CAD build for the part. Positions are in the model's coordinates, mm. Round coordinates to 2 decimals unless told otherwise and drop trailing zeros. Order: outer loops, then holes, each group sorted by start corner. A loop starts at its lowest first (then second) coordinate and runs counter-clockwise, first axis right, second up. Notation, with made-up numbers: (82, -24.75) -> (104, -24.75) arc R24 cw to (104, -1.75) -> close; hole circle Ø4 at (42.25, -7). An arc over 180 degrees is marked (long way). Return JSON: item names as keys, results as strings. Group by question number.
Q1. Cut at A-A (y = -1.75). Write the cut outline in (x, z).
Q2. Flat gauge pins, fed straight in: pin 1 (1 mm diameter, centred on x = -24.5, y = -3, fed in from +Z); pin 2 (3 mm diameter, centred on y = -1, z = -44, fed in from +X); pin 3 (2 mm diameter, centred on y = -1.5, z = -33.5, fed in from +X). Where does each tip first touch, or does it go through?
Q3. Cut at B-B (x = 3). Write the cut outline in (y, z), then the cut area to 3 significant figures.
Q4. Probe line 1 along Z through (x, y) = (-34, -1.55); line 2 along Z through (x, y) = (-46, -2); line 3 along X through (y, z) = (-1.75, 66.5). List the from-to ranges inside material, lowest first.
from build123d import *

# Parameters (mm, degrees)
F0_W     = 152.4
F0_H     = 152.4
F1_DEPTH = 5.08
F3_DEPTH = 5.08
F4_DEPTH = 25.4


with BuildPart() as f1:
    # F0 (on Front) → F1 (new body)
    with BuildSketch(Plane.XZ):
        with Locations((-57.4968958794, 22.0549479127)):
            Rectangle(F0_W, F0_H)
    extrude(amount=F1_DEPTH)

    # F2 (on face) → F3 (cut)
    with BuildSketch(Plane.XZ.offset(5.08)):
        with BuildLine():
            Line((18.7031041206, 98.2549479127), (-133.6968958794, 98.2549479127))
            ThreePointArc((-133.6968958794, 98.2549479127), (-76.6827848193, 2.8690589728), (18.7031041206, -54.1450520873))
            Line((18.7031041206, -54.1450520873), (18.7031041206, 98.2549479127))
        make_face()
    extrude(amount=-F3_DEPTH, mode=Mode.SUBTRACT)

    # F4 (add): a face of the model
    f4_faces = [f1.faces().sort_by_distance(p)[0] for p in [
        (-57.4968958794, -2.54, -54.1450520873),
    ]]
    extrude(f4_faces, amount=F4_DEPTH)


solid = f1.part
Solution:
{
 "1": {"outline": "(-133.7, -79.55) -> (18.7, -79.55) -> (18.7, -54.15) arc R227.57 cw to (-133.7, 98.25) -> close"},
 "2": {"pin 1": "stops at z = -35.85", "pin 2": "stops at x = -5.14", "pin 3": "stops at x = -27.44"},
 "3": {"outline": "(-5.08, -79.55) -> (0, -79.55) -> (0, -48.79) -> (-5.08, -48.79) -> close", "area": "156 mm²"},
 "4": {"line 1": "z = -79.55 to -30.66", "line 2": "z = -79.55 to -22.84", "line 3": "x = -133.7 to -121.49"}
}
